CAD build for the part. Positions are in the model's coordinates, mm. A direction names the side the tool comes from. Coordinates: 2 decimals unless noted, no trailing zeros. Order: outer loops, then holes, each group sorted by start corner. A loop starts at its lowest first (then second) coordinate and runs counter-clockwise, first axis right, second up. Notation, with made-up numbers: (21, -14) -> (66, -14) arc R7 cw to (66, -2) -> close; hole circle Ø7 at (36.5, 36). An arc over 180 degrees is marked (long way). Use one line per item in the form item = value. Start each with the question number.
from build123d import *

# Parameters (mm, degrees)
F1_DEPTH = 63.5
F2_DEPTH = 25.4
F3_DEPTH = 9.525


with BuildPart() as f1:
    # F0 (on Front) → F1 (new body, symmetric)
    with BuildSketch(Plane.XZ):
        Polygon((-41.275, -9.525), (41.275, -9.525), (41.275, 9.525), (22.225, 9.525), (-41.275, 9.525), align=None)
    extrude(amount=F1_DEPTH, both=True)

    # F0 (on Front) → F2 (join, symmetric)
    with BuildSketch(Plane.XZ):
        with BuildLine():
            Line((22.225, 9.525), (41.275, 9.525))
            Line((41.275, 9.525), (41.275, 36.5252))
            ThreePointArc((41.275, 36.5252), (45.92468, 47.75052), (57.15, 52.4002))
            Line((57.15, 52.4002), (60.325, 52.4002))
            Line((60.325, 52.4002), (60.325, 71.4502))
            Line((60.325, 71.4502), (57.15, 71.4502))
            add(Edge.make_bspline(
                [(49.751271, 70.657508), (52.166771, 70.942003), (54.632844, 71.205798), (57.15, 71.4502)],
                knots=[111.1633, 111.1633, 111.1633, 111.1633, 116.285042, 116.285042, 116.285042, 116.285042], degree=3))
            ThreePointArc((49.751271, 70.657508), (29.964009, 58.449559), (22.225, 36.5252))
            Line((22.225, 36.5252), (22.225, 9.525))
        make_face()
    extrude(amount=F2_DEPTH, both=True)

    # F0 (on Front) → F3 (join, symmetric)
    with BuildSketch(Plane.XZ):
        with BuildLine():
            add(Edge.make_bspline(
                [(-41.275, 9.525), (-31.278197, 48.557062), (-2.675208, 64.482776), (49.751271, 70.657508)],
                knots=[0, 0, 0, 0, 111.1633, 111.1633, 111.1633, 111.1633], degree=3))
            Line((-41.275, 9.525), (22.225, 9.525))
            Line((22.225, 9.525), (22.225, 36.5252))
            ThreePointArc((22.225, 36.5252), (29.964009, 58.449559), (49.751271, 70.657508))
        make_face()
    extrude(amount=F3_DEPTH, both=True)


solid = f1.part
1) Cut at A-A on y = 37. Give the cut face in (x, z) (3 decimals), then the cut area to 3 significant figures.
2) Cut at B-B on z = 3. Give the cut face in (x, y) (3 decimals).
3) 3-axis set-ups, long thin cutter, end or side, ignore diameter. For faces 1 (the face through (22.225, -18, 23)), 2 (the face through (37, -25.4, 41)), 3 (the face through (30.174, 17.351, 58.707)), 4 (the face through (37, 25.4, 41)), 5 (the face through (59, 0, 52.4)): which of +Z, -Z, +X, -X, +Y, -Y reach the whole face in a straight line?
4) Probe L1, parallel to Z at x = -15, y = -51 (3 decimals); L2, parallel to Y at x = 46.5, z = 62. List the from-to ranges inside material, lowest first.
5) Drop flat-ended pins along their axis: P1, Ø19, axis at x = 42, z = 41, coming from the -Y side; P2, Ø1.6, axis at x = 59, y = 6.5, coming from the -Z side; P3, Ø17.5, axis at y = 19.5, z = 21.5, coming from the -X side (3 decimals). Give the stop position or say it passes through.
Values follow:
q1.outline = (-41.275, -9.525) -> (41.275, -9.525) -> (41.275, 9.525) -> (-41.275, 9.525) -> close
q1.area = 1,570 mm^2
q2.outline = (-41.275, -63.5) -> (41.275, -63.5) -> (41.275, 63.5) -> (-41.275, 63.5) -> close
q3.face_1 = +Z, -X, -Y
q3.face_2 = +Z, +X, -X, -Y
q3.face_3 = +Z, -X, +Y
q3.face_4 = +Z, +X, -X, +Y
q3.face_5 = -Z, +X, +Y, -Y
q4.L1 = -9.525 to 9.525
q4.L2 = -25.4 to 25.4
q5.P1 = -25.4
q5.P2 = 52.4
q5.P3 = 22.225
